Autodesk Inventor part; units mm, degrees
ref_plane "YZ Plane" through (0, 0, 0) normal (1, 0, 0) x (0, 1, 0)
ref_plane "XZ Plane" through (0, 0, 0) normal (0, 1, 0) x (-1, 0, 0)
ref_plane "XY Plane" through (0, 0, 0) normal (0, 0, 1) x (1, 0, 0)
sketch "main" plane through (0, 0, 0) normal (0, 0, 1) x (1, 0, 0)
  line L0 (-3.1973, -8.3156) -> (0.4095, -8.3156)
  arc A0 (-3.1973, -8.3156) -> (-3.7053, -8.8236) centre (-3.1973, -8.8236) ccw
  arc A1 (0.9175, -8.8236) -> (0.4095, -8.3156) centre (0.4095, -8.8236) ccw
  line L1 (-3.7053, -12.4304) -> (-3.7053, -8.8236)
  line L2 (0.9175, -8.8236) -> (0.9175, -12.4304)
  arc A2 (-3.7053, -12.4304) -> (-3.1973, -12.9384) centre (-3.1973, -12.4304) ccw
  line L3 (0.4095, -12.9384) -> (-3.1973, -12.9384)
  arc A3 (0.4095, -12.9384) -> (0.9175, -12.4304) centre (0.4095, -12.4304) ccw
  spline S0 degree 3 poles (4.1061, -10.627) (4.1061, -11.3073) (4.0733, -12.6645) (2.9205, -14.6469) (1.3832, -15.5703) (0.4113, -15.8334) (0.0836, -15.9248) knots 0 0 0 0 0.294694 0.589389 0.884083 1.03143 1.03143 1.03143 1.03143
  arc A4 (-10.9164, -7.5728) -> (-6.8939, -2.275) centre (-12.3939, -2.275) ccw
  line L4 (-13.7381, -19.7795) -> (0.0836, -15.9248)
  line L5 (-10.9164, -7.5728) -> (-16.6931, -9.1839)
  arc A5 (-16.6931, -9.1839) -> (-13.7381, -19.7795) centre (-15.2156, -14.4817) ccw
  circle A6 centre (-15.2156, -14.4817) radius 2.1
  line L6 (0.4095, -0.2384) -> (-3.1973, -0.2384)
  arc A7 (-3.7053, 0.2696) -> (-3.1973, -0.2384) centre (-3.1973, 0.2696) ccw
  line L7 (0.9175, 3.8764) -> (0.9175, 0.2696)
  line L8 (-3.7053, 0.2696) -> (-3.7053, 3.8764)
  line L9 (-3.1973, 4.3844) -> (0.4095, 4.3844)
  arc A8 (-3.1973, 4.3844) -> (-3.7053, 3.8764) centre (-3.1973, 3.8764) ccw
  arc A9 (0.9175, 3.8764) -> (0.4095, 4.3844) centre (0.4095, 3.8764) ccw
  arc A10 (0.4095, -0.2384) -> (0.9175, 0.2696) centre (0.4095, 0.2696) ccw
  line L10 (4.1061, -10.627) -> (4.1061, 14.773)
  arc A11 (4.1061, 14.773) -> (-6.8939, 14.773) centre (-1.3939, 14.773) ccw
  line L11 (-6.8939, 14.773) -> (-6.8939, -2.275)
  line L12 (0.4095, 12.4616) -> (-3.1973, 12.4616)
  arc A12 (0.4095, 12.4616) -> (0.9175, 12.9696) centre (0.4095, 12.9696) ccw
  arc A13 (-3.7053, 12.9696) -> (-3.1973, 12.4616) centre (-3.1973, 12.9696) ccw
  line L13 (0.9175, 16.5764) -> (0.9175, 12.9696)
  line L14 (-3.7053, 12.9696) -> (-3.7053, 16.5764)
  arc A14 (-3.1973, 17.0844) -> (-3.7053, 16.5764) centre (-3.1973, 16.5764) ccw
  arc A15 (0.9175, 16.5764) -> (0.4095, 17.0844) centre (0.4095, 16.5764) ccw
  line L15 (-3.1973, 17.0844) -> (0.4095, 17.0844)
  point P0 (-2.9609, 0.4438)
  point P1 (-20.5005, 14.8552)
sketch "Sketch1" plane through (0, 0, 0) normal (0, 1, 0) x (-1, 0, 0)
  line L0 (-1.8034, -23.0886) -> (1.8034, -23.0886)
  arc A0 (-1.8034, -23.0886) -> (-2.3114, -23.5966) centre (-1.8034, -23.5966) ccw
  arc A1 (2.3114, -23.5966) -> (1.8034, -23.0886) centre (1.8034, -23.5966) ccw
  line L1 (-2.3114, -27.2034) -> (-2.3114, -23.5966)
  line L2 (2.3114, -23.5966) -> (2.3114, -27.2034)
  arc A2 (-2.3114, -27.2034) -> (-1.8034, -27.7114) centre (-1.8034, -27.2034) ccw
  line L3 (1.8034, -27.7114) -> (-1.8034, -27.7114)
  arc A3 (1.8034, -27.7114) -> (2.3114, -27.2034) centre (1.8034, -27.2034) ccw
  spline S0 degree 3 poles (5.5, -25.4) (5.5, -26.0803) (5.4672, -27.4376) (4.3143, -29.4199) (2.7771, -30.3433) (1.8052, -30.6064) (1.4775, -30.6978) knots 0 0 0 0 0.294694 0.589389 0.884083 1.03143 1.03143 1.03143 1.03143
  arc A4 (-9.5225, -22.3458) -> (-5.5, -17.048) centre (-11, -17.048) ccw
  line L4 (-12.3443, -34.5525) -> (1.4775, -30.6978)
  line L5 (-9.5225, -22.3458) -> (-15.2992, -23.9569)
  arc A5 (-15.2992, -23.9569) -> (-12.3443, -34.5525) centre (-13.8217, -29.2547) ccw
  circle A6 centre (-13.8217, -29.2547) radius 2.1
  line L6 (1.8034, -15.0114) -> (-1.8034, -15.0114)
  arc A7 (-2.3114, -14.5034) -> (-1.8034, -15.0114) centre (-1.8034, -14.5034) ccw
  line L7 (2.3114, -10.8966) -> (2.3114, -14.5034)
  line L8 (-2.3114, -14.5034) -> (-2.3114, -10.8966)
  line L9 (-1.8034, -10.3886) -> (1.8034, -10.3886)
  arc A8 (-1.8034, -10.3886) -> (-2.3114, -10.8966) centre (-1.8034, -10.8966) ccw
  arc A9 (2.3114, -10.8966) -> (1.8034, -10.3886) centre (1.8034, -10.8966) ccw
  arc A10 (1.8034, -15.0114) -> (2.3114, -14.5034) centre (1.8034, -14.5034) ccw
  line L10 (5.5, -25.4) -> (5.5, 0)
  arc A11 (5.5, 0) -> (-5.5, 0) centre (0, 0) ccw
  line L11 (-5.5, 0) -> (-5.5, -17.048)
  line L12 (1.8034, -2.3114) -> (-1.8034, -2.3114)
  arc A12 (1.8034, -2.3114) -> (2.3114, -1.8034) centre (1.8034, -1.8034) ccw
  arc A13 (-2.3114, -1.8034) -> (-1.8034, -2.3114) centre (-1.8034, -1.8034) ccw
  line L13 (2.3114, 1.8034) -> (2.3114, -1.8034)
  line L14 (-2.3114, -1.8034) -> (-2.3114, 1.8034)
  arc A14 (-1.8034, 2.3114) -> (-2.3114, 1.8034) centre (-1.8034, 1.8034) ccw
  arc A15 (2.3114, 1.8034) -> (1.8034, 2.3114) centre (1.8034, 1.8034) ccw
  line L15 (-1.8034, 2.3114) -> (1.8034, 2.3114)
extrude "Extrusion1" add sketch "Sketch1" along normal blind 1.5875
properties part number "bent_gusset_nesting"
Here's how the part is built. I have some questions about the finished solid (model axes, mm). A direction names the side the tool comes from. Round coordinates to 2 decimals unless told otherwise and drop trailing zeros. Loops run counter-clockwise (first coordinate to the right, second up) from the corner with the lowest first, then second, coordinate; pieces in that order, holes last. Notation, with made-up numbers: M 74,70.5 L 126,70.5 A14 ccw 126,81.5 Z; hole C 84,-37 d9. An arc over 180 degrees is marked long. Write each question's results on one line, items separated by ' | '. Start each with the question number.
(1) I want a section at B-B (x = 0). Please give me the cut outline in (y, z).
(2) I want a section at D-D (y = 0.5). State how many separate pieces and enclosed holes the cut face has, then the cut area to 3 significant figures.
(3) I want a section at A-A (z = -14). Please give me the cut outline in (x, y), then the cut area to 3 significant figures.
(4) If I drill on probe 1 along Z at (x, y) = (-0.5, 1.15); probe 2 along X at (y, z) = (0.3, -14); probe 3 along X at (y, z) = (0.8, -26), over which ranges is the centre line in solid material (lowest first)? Write a range as from..to.
(5) Will these pins go through, and if not, where does the flat tip stop? P1, Ø0.5, axis at y = 1, z = -26, coming from the +X side; P2, Ø0.8, axis at x = 0.5, y = 1, coming from the -Z side; P3, Ø0.8, axis at y = 1, z = -7, coming from the +X side.
(6) On a 3-axis mill with a long thin cutter (end or side, diameter ignored), from which of +Z, -Z, +X, -X, +Y, -Y can I reach the whole of each face in a straight line? I mean faces 4 (the flat face through (0, 1, 2.311)), 5 (the flat face through (4, 1.588, -19)), 6 (the flat face through (5.5, 1, -8)). Say none if no direction works.
(7) I want a section at C-C (x = 12.75). Please give me the cut outline in (y, z), then the cut area to 3 significant figures.
(8) Thinking about a two-plate mould opening in Z: for faces 1 (the flat face through (5.53, 0.783, -32.652)), 2 (the cylindrical face through (14.277, 0.783, -27.205)), 3 (the cylindrical face through (0.1, 0.8, 5.5)), which applies, pulls with the +Z half, pulls with the -Z half, needs draft (parallel to the pull), parting line crosses it, or undercut?
Solved:
1) outline: M 0,-31.11 L 1.59,-31.11 L 1.59,-27.71 L 0,-27.71 Z; M 0,-23.09 L 1.59,-23.09 L 1.59,-15.01 L 0,-15.01 Z; M 0,-10.39 L 1.59,-10.39 L 1.59,-2.31 L 0,-2.31 Z; M 0,2.31 L 1.59,2.31 L 1.59,5.5 L 0,5.5 Z
2) separate pieces: 1 | enclosed holes: 4 | area: 456 mm²
3) outline: M -5.5,0 L -2.31,0 L -2.31,1.59 L -5.5,1.59 Z; M 2.31,0 L 5.5,0 L 5.5,1.59 L 2.31,1.59 Z | area: 10.1 mm²
4) probe 1: z = -30.97..-27.71, -23.09..-15.01, -10.39..-2.31, 2.31..5.48 | probe 2: x = -5.5..-2.31, 2.31..5.5 | probe 3: x = -5.49..-2.31, 2.31..18.26
5) P1: stops at x = 18.43 | P2: stops at z = -31.36 | P3: stops at x = 5.5
6) face 4: +Y, -Y | face 5: +Z, -Z, +X, -X, +Y | face 6: +Z, +X, +Y, -Y
7) outline: M 0,-34.65 L 1.59,-34.65 L 1.59,-31.06 L 0,-31.06 Z; M 0,-27.45 L 1.59,-27.45 L 1.59,-23.25 L 0,-23.25 Z | area: 12.4 mm²
8) face 1: pulls with the -Z half | face 2: undercut | face 3: pulls with the +Z half
